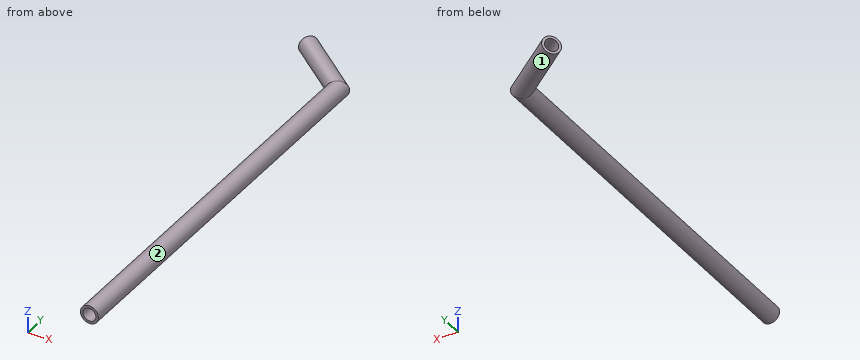
Autodesk Inventor part; units mm, degrees
ref_plane "YZ Plane" through (0, 0, 0) normal (1, 0, 0) x (0, 1, 0)
ref_plane "XZ Plane" through (0, 0, 0) normal (0, 1, 0) x (-1, 0, 0)
ref_plane "XY Plane" through (0, 0, 0) normal (0, 0, 1) x (1, 0, 0)
sketch "Sketch1" plane through (0, 0, 0) normal (0, 1, 0) x (-1, 0, 0)
  circle A0 centre (0, 0) radius 2.286
  circle A1 centre (0, 0) radius 3.175
  dimension "d0" = 4.572
  dimension "d1" = 6.35
sketch "Sketch2" plane through (0, 0, 0) normal (0, 0, 1) x (1, 0, 0)
  line L0 (0, 0) -> (0, 92.964)
  line L1 (0, 0) -> (92.964, 0) construction
  line L2 (0, 92.964) -> (0, 141.224)
  line L3 (0, 141.224) -> (-20.0427, 156.8268)
  line L4 (0, 141.224) -> (25.4, 141.224) construction
  dimension "d2" = 92.964
  dimension "d3" = 90
  dimension "d4" = 48.26
  dimension "d5" = 25.4
  dimension "d6" = 142.1
sweep "Sweep1" add profiles "Sketch1" path "Sketch2"
properties part number "feedthroughpipe"
Can you work these out from the model? Positions are in its coordinate system, mm. Face numbers are marked on the shaded views. A direction names the side the tool comes from. Round coordinates to 2 decimals unless told otherwise and drop trailing zeros. Write each loop counter-clockwise with the first axis right and the second up, starting at its lowest first coordinate (ties: lowest second). Pieces come first, ordered by that corner, then holes. Notation, with made-up numbers: (-30.5, 44.25) - (-13.5, 44.25) arc R10 cw to (-13.5, 50.25) - close; hole circle Ø10 at (42, 0.25). An arc over 180 degrees is marked (long way). Write each question's results on one line, items separated by ' | '. Start each with the question number.
1) Which directions (+Z, -Z, +X, -X, +Y, -Y) give clear straight access to the entire face, cutting with the end or side of a thin tool? Please do the marked faces 1 and 2.
2) Please list where these lines run through material, in increasing order: line 1 (Z direction, x = 0, y = 40) (3 decimals); line 2 (Y direction, x = -11.25, z = 1).
3) For pin 1 Ø10 at (x, y) = (-5.5, 40) entering from +Z; pin 2 Ø1 at (x, z) = (0, 1.5) entering from +Y; pin 3 Ø2 at (x, z) = (-15, -1) entering from +Y; pin 4 Ø5 at (x, y) = (-7.5, 108.5) entering from +Z, each with a flat end and sliding along its axis, tell me the tip position at first contact or that it passes through.
4) Suppose I cut it at A-A (z = 0). List the corners of the cut face in (x, y) for me (3 decimals), and give its area (3 significant figures).
5) Suppose I cut it at B-B (y = 27). List the corners of the cut face in (x, z) for me (3 decimals).
Here are the results:
1) face 1: none | face 2: -Y
2) line 1: z = -3.175 to -2.286, 2.286 to 3.175 | line 2: y = 146.16 to 147.38, 152.59 to 153.8
3) pin 1: stops at z = 3.14 | pin 2: stops at y = 145.26 | pin 3: stops at y = 157.57 | pin 4: passes through
4) outline: (-21.993, 154.321) - (-3.175, 139.672) - (-3.175, 0) - (-2.286, 0) - (-2.286, 140.107) - (-21.447, 155.023) - close; (-18.638, 158.631) - (2.286, 142.341) - (2.286, 0) - (3.175, 0) - (3.175, 142.776) - (-18.092, 159.332) - close | area: 296 mm2
5) outline: circle Ø6.35 at (0, 0); hole circle Ø4.572 at (0, 0)
